Geometry check sheet. Reference: the model listing, model coordinates, mm. Round coordinates to 2 decimals unless told otherwise and drop trailing zeros. Order: outer loops, then holes, each group sorted by start corner. A loop starts at its lowest first (then second) coordinate and runs counter-clockwise, first axis right, second up. Notation, with made-up numbers: (80, -34) - (137, -34) arc R35 cw to (137, 5) - close; hole circle Ø5 at (8, 39.5). An arc over 180 degrees is marked (long way). One line per question, with ' | ' between items. Start each with the question number.
Q1. Gauge pin test, flat end, axial feed: P1, Ø6, axis at x = 0, z = -21.24, coming from the +Y side. Record the tip position at first contact, or that the pin passes through.
Q2. Sectioned sample at B-B, the plane y = -2.75. Enter the section's corners in (x, z).
Q3. Material ranges on line 1 along Z through (x, y) = (0, -0.5); line 2 along Z through (x, y) = (2.25, -4.5); line 3 along Z through (x, y) = (5.25, -4.2), recorded low to high.
Q4. Mould release check, pull along Z, two halves, no side actions. Record for faces 1 (the face through (-0.661, -2.504, -16.208)), 2 (the face through (-6.35, -3, 30)), 3 (the face through (-0.14, -2.504, -27.593)): +Z half, -Z half, draft (parallel to the pull), parting line (faces both ways), or undercut.
Q5. Sectioned sample at A-A, the plane x = 0. Enter the section's corners in (y, z), then the cut area to 3 significant figures.
```python
from build123d import *

# Parameters (mm, degrees)
F0_R     = 5.08
F1_DEPTH = 5.08


with BuildPart() as f1:
    # F0 (on Front) → F1 (new body)
    with BuildSketch(Plane.XZ):
        with BuildLine():
            Line((6.35, -21.244763), (6.35, 80.355237))
            ThreePointArc((6.35, 80.355237), (0, 74.005237), (-6.35, 80.355237))
            Line((-6.35, 80.355237), (-6.35, -21.244763))
            ThreePointArc((-6.35, -21.244763), (0, -14.894763), (6.35, -21.244763))
        make_face()
        with BuildLine():
            ThreePointArc((-6.35, 80.355237), (0, 74.005237), (6.35, 80.355237))
            ThreePointArc((6.35, 80.355237), (0, 86.705237), (-6.35, 80.355237))
        make_face()
        with Locations((0, 80.355237)):
            Circle(F0_R, mode=Mode.SUBTRACT)
        with BuildLine():
            ThreePointArc((-6.35, -21.244763), (0, -27.594763), (6.35, -21.244763))
            ThreePointArc((6.35, -21.244763), (0, -14.894763), (-6.35, -21.244763))
        make_face()
        with Locations((0, -21.244763)):
            Circle(F0_R, mode=Mode.SUBTRACT)
    extrude(amount=F1_DEPTH)


solid = f1.part
```
Determined:
1) P1: passes through
2) outline: (-6.35, -21.24) arc R6.35 ccw to (6.35, -21.24) - (6.35, 80.36) arc R6.35 ccw to (-6.35, 80.36) - close; hole circle Ø10.16 at (0, -21.24); hole circle Ø10.16 at (0, 80.36)
3) line 1: z = -27.59 to -26.32, -16.16 to 75.28, 85.44 to 86.71 | line 2: z = -27.18 to -25.8, -16.69 to 75.8, 84.91 to 86.29 | line 3: z = -24.82 to 83.93
4) face 1: undercut | face 2: draft | face 3: -Z half
5) outline: (-5.08, -27.59) - (0, -27.59) - (0, -26.32) - (-5.08, -26.32) - close; (-5.08, -16.16) - (0, -16.16) - (0, 75.28) - (-5.08, 75.28) - close; (-5.08, 85.44) - (0, 85.44) - (0, 86.71) - (-5.08, 86.71) - close | area: 477 mm2
